from build123d import *

# Parameters (mm, degrees)
SKETCH_1_W      = 50
SKETCH_1_H      = 50
EXTRUDE_1_DEPTH = 4
SKETCH_2_R      = 10
EXTRUDE_2_DEPTH = 40
FILLET_1_R      = 10
FILLET_2_R      = 10
FILLET_3_R      = 10


with BuildPart() as part:
    # 草图1 → 凸台-拉伸1 (new body)
    with BuildSketch(Plane(origin=(0, 0, 0), x_dir=(1, 0, 0), z_dir=(0, 1, 0))):
        with Locations((25, -25)):
            Rectangle(SKETCH_1_W, SKETCH_1_H)
    extrude(amount=EXTRUDE_1_DEPTH)

    # 草图2 → 凸台-拉伸2 (add)
    with BuildSketch(Plane(origin=(0, 4, 0), x_dir=(1, 0, 0), z_dir=(0, 1, 0))):
        with Locations(Location((25, -25, 0), (0, 0, 270))):
            Circle(SKETCH_2_R)
    extrude(amount=EXTRUDE_2_DEPTH)

    # 圆角1
    fillet_1_edges = [part.edges().sort_by_distance(p)[0] for p in [
        (25, 4, 15),
    ]]
    fillet(fillet_1_edges, radius=FILLET_1_R)

    # 圆角2
    fillet_2_edges = [part.edges().sort_by_distance(p)[0] for p in [
        (25, 44, 15),
    ]]
    fillet(fillet_2_edges, radius=FILLET_2_R)

    # 圆角3
    fillet_3_edges = [part.edges().sort_by_distance(p)[0] for p in [
        (0, 2, 0),
        (50, 2, 0),
        (50, 2, 50),
        (0, 2, 50),
    ]]
    fillet(fillet_3_edges, radius=FILLET_3_R)


solid = part.part
Input: part model. Units: mm. Frame: model coordinates. A direction names the side the tool comes from. Give positions to 0.01 mm unless a question says otherwise; leave off trailing zeros. Order: outer loops, then holes, each group sorted by start corner. A loop starts at its lowest first (then second) coordinate and runs counter-clockwise, first axis right, second up. Notation, with made-up numbers: (52.5, 11) - (82.5, 11) arc R33 ccw to (82.5, 47) - close; hole circle Ø7 at (-37.75, 85.25). An arc over 180 degrees is marked (long way). Write each question's results on one line, items separated by ' | '.
Item 1: Section A-A (z = 25). Return loops of the section in (x, y).
A:
outline: (0, 0) - (50, 0) - (50, 4) - (45, 4) arc R10 cw to (35, 14) - (35, 34) arc R10 ccw to (15, 34) - (15, 14) arc R10 cw to (5, 4) - (0, 4) - close
Item 2: Section D-D (y = 35). Return loops of the section in (x, z), and give its area (3 significant figures).
A:
outline: circle Ø19.9 at (25, 25) | area: 311 mm^2
Item 3: Material intervals for line 1 along Y through (x, z) = (45.5, 18); line 2 along X through (y, z) = (8, 24.5); line 3 along Z through (x, y) = (27.5, 32.5), sorted ascending.
A:
line 1: y = 0 to 4 | line 2: x = 13.01 to 36.99 | line 3: z = 15.32 to 34.68
Item 4: Access query for faces 1 (the flat face through (14, 4, 8)), 2 (the flat face through (25, 2, 0)). Directions: +Z, -Z, +X, -X, +Y, -Y. A direction counts if a zero-diameter tool reaches every point of the face in a straight line with its end or side. Return the directions, or none.
A:
face 1: +Y | face 2: -Z, +X, -X, +Y, -Y
Item 5: Section B-B (x = 25). Return loops of the section in (y, z), and give its area (3 significant figures).
A:
outline: (0, 0) - (4, 0) - (4, 5) arc R10 cw to (14, 15) - (34, 15) arc R10 ccw to (34, 35) - (14, 35) arc R10 cw to (4, 45) - (4, 50) - (0, 50) - close | area: 1,000 mm^2
Item 6: Section C-C (y = 17). Return loops of the section in (x, z).
A:
outline: circle Ø20 at (25, 25)
Item 7: Contact query for flat-ended pins moving along their axis: pin 1 Ø1 at (y, z) = (11, 24) entering from +X; pin 2 Ø5 at (x, y) = (14, 21) entering from -Z; pin 3 Ø5 at (x, y) = (26, 23) entering from -Z. Output: stop coordinate, or through.
A:
pin 1: stops at x = 35.59 | pin 2: stops at z = 19.73 | pin 3: stops at z = 15
